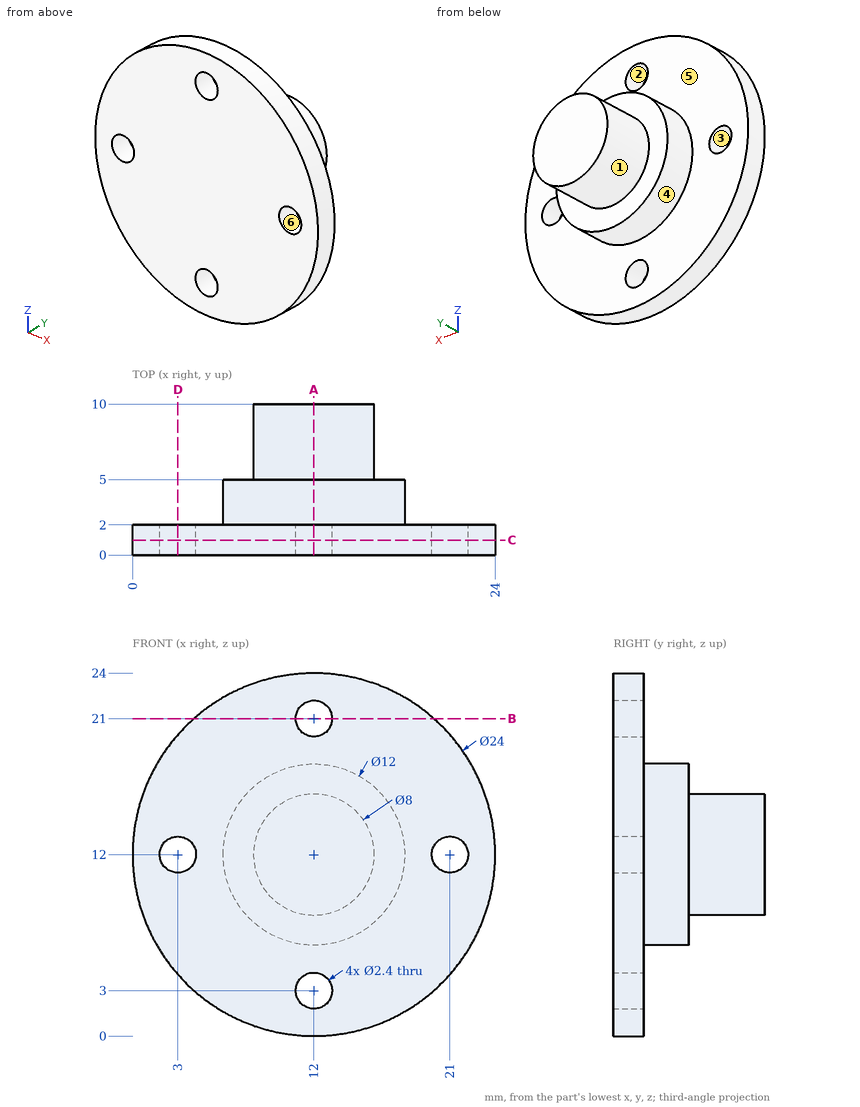
Check sheet for the drawn part. Datum: minimum x, y, z corner. Units: mm. A direction names the side the tool comes from. Round coordinates to 2 decimals unless told otherwise and drop trailing zeros. Loops run counter-clockwise (first coordinate to the right, second up) from the corner with the lowest first, then second, coordinate; pieces in that order, holes last. Notation, with made-up numbers: (18.5, 7) -> (72.5, 7) arc R24 cw to (72.5, 24) -> close; hole circle Ø8 at (54.5, 39.25). An arc over 180 degrees is marked (long way). Put each result on its own line as item: value. Start each with the question number.
1. Section check A-A (x = 12). Enter the section's corners in (y, z).
2. Section check D-D (x = 3). Enter the section's corners in (y, z).
3. Draft check along Z on the marked faces 3, 4, 5 and 6. Enter one of: +Z half, -Z half, draft (parallel to the pull), parting line (faces both ways), or undercut.
4. Scan lines: probe 1 along Z at (x, y) = (12, 0.65); probe 2 along Y at (x, z) = (2, 16); probe 3 along Z at (x, y) = (21, 1.3). Record each from-to range of solid material in increasing order.
5. Access from +Z, -Z, +X, -X, +Y, -Y to the whole of each face (thin tool, end or side, straight path). Record for the marked faces 1 and 2.
6. Section check C-C (y = 1). Enter the section's corners in (x, z).
7. Section check B-B (z = 21). Enter the section's corners in (x, y).
8. Gauge pin test, flat ends, axial feed: pin 1 (1 mm diameter, centred on x = 9, z = 8, fed in from +Y); pin 2 (1.5 mm diameter, centred on x = 20, z = 19, fed in from +Y); pin 3 (1.5 mm diameter, centred on y = 7, z = 15.5, fed in from +X). Record the tip position at first contact, or that the pin passes through.
Findings:
1. outline: (0, 0) -> (2, 0) -> (2, 1.8) -> (0, 1.8) -> close; (0, 4.2) -> (2, 4.2) -> (2, 6) -> (5, 6) -> (5, 8) -> (10, 8) -> (10, 16) -> (5, 16) -> (5, 18) -> (2, 18) -> (2, 19.8) -> (0, 19.8) -> close; (0, 22.2) -> (2, 22.2) -> (2, 24) -> (0, 24) -> close
2. outline: (0, 4.06) -> (2, 4.06) -> (2, 10.8) -> (0, 10.8) -> close; (0, 13.2) -> (2, 13.2) -> (2, 19.94) -> (0, 19.94) -> close
3. face 3: undercut
3. face 4: parting line
3. face 5: draft
3. face 6: undercut
4. probe 1: z = 0 to 1.8, 4.2 to 19.8, 22.2 to 24
4. probe 2: y = 0 to 2
4. probe 3: z = 4.06 to 10.8, 13.2 to 19.94
5. face 1: +Y
5. face 2: +Y, -Y
6. outline: circle Ø24 at (12, 12); hole circle Ø2.4 at (3, 12); hole circle Ø2.4 at (12, 3); hole circle Ø2.4 at (12, 21); hole circle Ø2.4 at (21, 12)
7. outline: (4.06, 0) -> (10.8, 0) -> (10.8, 2) -> (4.06, 2) -> close; (13.2, 0) -> (19.94, 0) -> (19.94, 2) -> (13.2, 2) -> close
8. pin 1: stops at y = 5
8. pin 2: stops at y = 2
8. pin 3: stops at x = 14.9
